Can you work these out from the model? Positions are in its coordinate system, mm. A direction names the side the tool comes from. Coordinates: 2 decimals unless noted, no trailing zeros. Order: outer loops, then holes, each group sorted by start corner. A loop starts at its lowest first (then second) coordinate and runs counter-clockwise, first axis right, second up. Notation, with made-up numbers: M 30.25,-12.5 L 48.25,-12.5 A24 ccw 48.25,11.5 Z; hole C 83.5,23.25 d9. An arc over 180 degrees is marked long. Answer as a JSON object with one key per item and string values.
from build123d import *

# Parameters (mm, degrees)
F0_W     = 25
F0_H     = 34.8
F1_DEPTH = 12.5
F3_START = -2.2
F2_R     = 10.35
F3_DEPTH = 30.4
F4_W     = 20.7
F4_H     = 1.52
F5_DEPTH = 10.6
F6_R     = 5
F7_R     = 2
F8_R     = 1.5
F9_DEPTH = 2.5


with BuildPart() as f1:
    # F0 (on Top) → F1 (new body)
    with BuildSketch(Plane.XY):
        with Locations((-17.5982150249, -9.7193448131)):
            Rectangle(F0_W, F0_H)
    extrude(amount=F1_DEPTH)

    # F2 (on face) → F3 (cut)
    with BuildSketch(Plane.XZ.offset(27.1193448131).offset(F3_START)):
        with Locations((-17.5982150249, 12.5)):
            Circle(F2_R)
    extrude(amount=-F3_DEPTH, mode=Mode.SUBTRACT)

    # F4 (on face) → F5 (join)
    with BuildSketch(Plane.XY.offset(12.5)):
        with Locations((-17.5982150249, 0.9206551869)):
            Rectangle(F4_W, F4_H)
        with Locations((-17.5982150249, -4.3993448131)):
            Rectangle(F4_W, F4_H)
        with Locations((-17.5982150249, -9.7193448131)):
            Rectangle(F4_W, F4_H)
        with Locations((-17.5982150249, -15.0393448131)):
            Rectangle(F4_W, F4_H)
        with Locations((-17.5982150249, -20.3593448131)):
            Rectangle(F4_W, F4_H)
    extrude(amount=-F5_DEPTH)

    # F6
    f6_edges = [f1.edges().sort_by_distance(p)[0] for p in [
        (-5.098215, -9.719345, 0),
        (-30.098215, -9.719345, 0),
    ]]
    fillet(f6_edges, radius=F6_R)

    # F7
    f7_edges = [f1.edges().sort_by_distance(p)[0] for p in [
        (-5.098215, -27.119345, 8.75),
        (-5.098215, 7.680655, 8.75),
    ]]
    fillet(f7_edges, radius=F7_R)

    # F8 (on face) → F9 (cut)
    with BuildSketch(Plane.XY.offset(12.5)):
        with Locations((-30.0982150249, 0.9206551869)):
            Circle(F8_R)
        with Locations((-5.0982150249, 0.9206551869)):
            Circle(F8_R)
        with Locations((-5.0982150249, -20.3593448131)):
            Circle(F8_R)
        with Locations((-30.0982150249, -20.3593448131)):
            Circle(F8_R)
    extrude(amount=-F9_DEPTH, mode=Mode.SUBTRACT)


solid = f1.part
Item 1: If we mould it in two halves opening along X, with no side actions, what happens to faces 1 (the cylindrical face through (-29.497, 7.11, 8.698)), 2 (the flat face through (-18, -8.959, 9)), 3 (the cylindrical face through (-17.49, -26.55, 0.6))? For each: pulls with the +X half, pulls with the -X half, needs draft (parallel to the pull), parting line crosses it, or undercut.
Answers follow:
{"face 1": "pulls with the -X half", "face 2": "undercut", "face 3": "needs draft"}
Item 2: Which directions (+Z, -Z, +X, -X, +Y, -Y) give clear straight access to the entire face, cutting with the end or side of a thin tool? Please do faces 4 (the flat face through (-6, -20, 10)), 5 (the flat face through (-29.5, 0.9, 10)), 6 (the flat face through (-18, -15.799, 9)), 7 (the cylindrical face through (-29.497, -26.549, 8.698)), 8 (the flat face through (-18, -10, 0)).
Answers follow:
{"face 4": "+Z, +X", "face 5": "+Z, -X", "face 6": "+Z", "face 7": "+Z, -Z, -X, -Y", "face 8": "-Z, +X, -X, +Y, -Y"}
Item 3: I want a section at C-C, the plane z = 11.5. Give the number of separate pieces and of enclosed holes in the cut face, plus the area to 3 significant figures.
Answers follow:
{"separate pieces": "1", "enclosed holes": "6", "area": "383 mm^2"}
Item 4: Please list where these lines run through material, in increasing order: line 1 (X direction, y = 2.5, z = 12.25); line 2 (X direction, y = -12, z = 3.25); line 3 (Z direction, x = -11.5, y = -21.5).
Answers follow:
{"line 1": "x = -30.1 to -27.95, -7.25 to -5.1", "line 2": "x = -29.78 to -22.24, -12.95 to -5.41", "line 3": "z = 0 to 4.14"}
Item 5: I want a section at A-A, the plane y = -8.5. Write out the boundary of the cut face in (x, z).
Answers follow:
{"outline": "M -30.1,5 A5 ccw -25.1,0 L -10.1,0 A5 ccw -5.1,5 L -5.1,12.5 L -7.25,12.5 A10.35 cw -27.95,12.5 L -30.1,12.5 Z"}
Item 6: I'm going to push a flat-ended pin straight in: pin 1 (0.8 mm diameter, centred on x = -5.5, y = -20.5, fed in from +Z). Where does the tip first touch, or does it pass through?
Answers follow:
{"pin 1": "stops at z = 10"}
